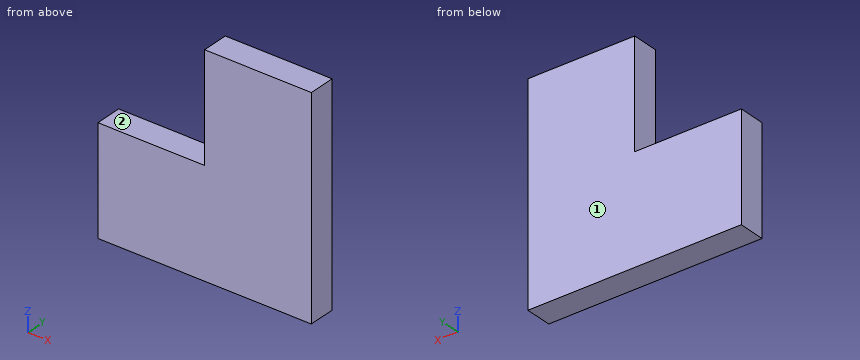
```python
from build123d import *

# Parameters (mm, degrees)
SKETCH1_W           = 100
SKETCH1_H           = 100
SKETCH1_W_2         = 200
BOSS_EXTRUDE1_DEPTH = 25


with BuildPart() as part:
    # Sketch1 → Boss-Extrude1 (new body)
    with BuildSketch(Plane(origin=(0, 0, 0), x_dir=(1, 0, 0), z_dir=(0, 1, 0))):
        with Locations((50, -100)):
            Rectangle(SKETCH1_W, SKETCH1_H)
        Rectangle(SKETCH1_W_2, SKETCH1_H)
    extrude(amount=BOSS_EXTRUDE1_DEPTH)


solid = part.part
```
Read the model definition and answer for the solid it produces. Units are mm, in the model's axes. Face numbers are marked on the shaded views. A direction names the side the tool comes from. Coordinates: 2 decimals unless noted, no trailing zeros. Loops run counter-clockwise (first coordinate to the right, second up) from the corner with the lowest first, then second, coordinate; pieces in that order, holes last. Notation, with made-up numbers: (81, 3.25) -> (90, 3.25) arc R22 ccw to (90, 22.25) -> close; hole circle Ø9 at (58.5, 29.5). An arc over 180 degrees is marked (long way). Return JSON: item names as keys, results as strings.
Item 1: Flat-ended cylindrical pins translate along their axes: P1, Ø6, axis at x = -47.5, y = 18, coming from the +Z side; P2, Ø6, axis at y = 15, z = 55.5, coming from the -X side. Find the tip coordinate at first contact, or state that the pin passes through.
Answers:
{"P1": "stops at z = 50", "P2": "stops at x = 0"}
Item 2: For the marked faces 1 and 2, determine the directions among +Z, -Z, +X, -X, +Y, -Y from which every point of the face is accessible in a straight line to the end or side of a thin tool.
Answers:
{"face 1": "+Z, -Z, +X, -X, +Y", "face 2": "+Z, -X, +Y, -Y"}
Item 3: Find section B-B (z = 58). Determine the outline of the cut face in (x, y), plus the area to 3 significant figures.
Answers:
{"outline": "(0, 0) -> (100, 0) -> (100, 25) -> (0, 25) -> close", "area": "2,500 mm2"}
Item 4: Find section A-A (y = 15). Determine the outline of the cut face in (x, z), plus the area to 3 significant figures.
Answers:
{"outline": "(-100, -50) -> (100, -50) -> (100, 150) -> (0, 150) -> (0, 50) -> (-100, 50) -> close", "area": "30,000 mm2"}
Item 5: Find the intervals of material crossed by probe 1 along X at (y, z) = (21.25, 59.5); probe 2 along Z at (x, y) = (-2.5, 22.25), in increasing order.
Answers:
{"probe 1": "x = 0 to 100", "probe 2": "z = -50 to 50"}
